from build123d import *

# Parameters (mm, degrees)
SKETCH1_W           = 47
SKETCH1_H           = 23.6
SKETCH1_W_2         = 44.18
SKETCH1_H_2         = 19
BOSS_EXTRUDE1_DEPTH = 5.5
SKETCH3_W           = 44.18
SKETCH3_H           = 19
BOSS_EXTRUDE2_DEPTH = 3
SKETCH6_W           = 7.25
SKETCH6_H           = 5.5
BOSS_EXTRUDE3_DEPTH = 5.25
SKETCH7_W           = 7.25
SKETCH7_H           = 5.5
BOSS_EXTRUDE4_DEPTH = 5.25
SKETCH8_R           = 1.5
CUT_EXTRUDE2_DEPTH  = 6.5
SKETCH9_W           = 51.734881385
SKETCH9_H           = 36.74917656
CUT_EXTRUDE3_DEPTH  = 3
SKETCH10_W          = 1.41
SKETCH10_H          = 14
BOSS_EXTRUDE5_DEPTH = 4
SKETCH11_W          = 3
SKETCH11_H          = 2.5
BOSS_EXTRUDE6_DEPTH = 3
SKETCH12_W          = 1.41
SKETCH12_H          = 8
CUT_EXTRUDE4_DEPTH  = 3.6
FILLET1_R           = 0.7


with BuildPart() as part:
    # Sketch1 → Boss-Extrude1 (new body)
    with BuildSketch(Plane(origin=(0, 0, 0), x_dir=(1, 0, 0), z_dir=(0, 1, 0))):
        with Locations((22.09, 9.5)):
            Rectangle(SKETCH1_W, SKETCH1_H)
        with Locations((22.09, 9.5)):
            Rectangle(SKETCH1_W_2, SKETCH1_H_2, mode=Mode.SUBTRACT)
    extrude(amount=BOSS_EXTRUDE1_DEPTH)

    # Sketch3 → Boss-Extrude2 (add)
    with BuildSketch(Plane.XZ):
        with Locations((22.09, -9.5)):
            Rectangle(SKETCH3_W, SKETCH3_H)
    extrude(amount=-BOSS_EXTRUDE2_DEPTH)

    # Sketch6 → Boss-Extrude3 (add)
    with BuildSketch(Plane.XY.offset(2.3)):
        with Locations((2.215, 2.75)):
            Rectangle(SKETCH6_W, SKETCH6_H)
        with Locations((41.965, 2.75)):
            Rectangle(SKETCH6_W, SKETCH6_H)
    extrude(amount=BOSS_EXTRUDE3_DEPTH)

    # Sketch7 → Boss-Extrude4 (add)
    with BuildSketch(Plane(origin=(0, 0, -21.3), x_dir=(-1, 0, 0), z_dir=(0, 0, -1))):
        with Locations((-41.965, 2.75)):
            Rectangle(SKETCH7_W, SKETCH7_H)
        with Locations((-2.215, 2.75)):
            Rectangle(SKETCH7_W, SKETCH7_H)
    extrude(amount=BOSS_EXTRUDE4_DEPTH)

    # Sketch8 → Cut-Extrude2 (cut, through all)
    with BuildSketch(Plane(origin=(0, 5.5, 0), x_dir=(1, 0, 0), z_dir=(0, 1, 0))):
        with Locations((41.965, 22.925)):
            Circle(SKETCH8_R)
        with Locations((41.965, -3.925)):
            Circle(SKETCH8_R)
        with Locations((2.215, -3.925)):
            Circle(SKETCH8_R)
        with Locations((2.215, 22.925)):
            Circle(SKETCH8_R)
    extrude(amount=-CUT_EXTRUDE2_DEPTH, mode=Mode.SUBTRACT)

    # Sketch9 → Cut-Extrude3 (cut)
    with BuildSketch(Plane.XZ):
        with Locations((23.178173587, -9.700906739)):
            Rectangle(SKETCH9_W, SKETCH9_H)
    extrude(amount=-CUT_EXTRUDE3_DEPTH, mode=Mode.SUBTRACT)

    # Sketch10 → Boss-Extrude5 (add)
    with BuildSketch(Plane(origin=(0, 5.5, 0), x_dir=(1, 0, 0), z_dir=(0, 1, 0))):
        with Locations((-0.705, 9.5)):
            Rectangle(SKETCH10_W, SKETCH10_H)
    extrude(amount=BOSS_EXTRUDE5_DEPTH)

    # Sketch11 → Boss-Extrude6 (add)
    with BuildSketch(Plane.ZY.offset(-44.18)):
        with Locations((-17.5, 4.25)):
            Rectangle(SKETCH11_W, SKETCH11_H)
        with Locations((-1.5, 4.25)):
            Rectangle(SKETCH11_W, SKETCH11_H)
    extrude(amount=BOSS_EXTRUDE6_DEPTH)

    # Sketch12 → Cut-Extrude4 (cut)
    with BuildSketch(Plane.XZ.offset(-3)):
        with Locations((-0.705, -9.5)):
            Rectangle(SKETCH12_W, SKETCH12_H)
    extrude(amount=-CUT_EXTRUDE4_DEPTH, mode=Mode.SUBTRACT)

    # Fillet1
    fillet1_edges = [part.edges().sort_by_distance(p)[0] for p in [
        (45.59, 5.5, -9.5),
        (0, 5.5, -17.75),
        (-1.41, 5.5, 2.525),
        (0, 5.5, -1.25),
        (20.59, 5.5, 0),
        (-1.41, 7.5, -16.5),
        (-0.705, 5.5, -2.5),
        (-1.41, 7.5, -2.5),
        (0, 7.5, -2.5),
        (-0.705, 5.5, -16.5),
        (0, 7.5, -16.5),
        (20.59, 5.5, -19),
        (42.68, 5.5, -16),
        (41.18, 5.5, -17.5),
        (44.18, 5.5, -9.5),
        (42.68, 5.5, -3),
        (41.18, 5.5, -1.5),
        (-1.41, 5.5, -21.525),
        (22.09, 5.5, 2.3),
        (5.84, 5.5, 4.925),
        (2.215, 5.5, 7.55),
        (38.34, 5.5, 4.925),
        (41.965, 5.5, 7.55),
        (22.09, 5.5, -21.3),
        (38.34, 5.5, -23.925),
        (41.965, 5.5, -26.55),
        (5.84, 5.5, -23.925),
        (2.215, 5.5, -26.55),
    ]]
    fillet(fillet1_edges, radius=FILLET1_R)


solid = part.part
Input: part model. Units: mm. Frame: model coordinates. A direction names the side the tool comes from. Give positions to 0.01 mm unless a question says otherwise; leave off trailing zeros. Write each loop counter-clockwise with the first axis right and the second up, starting at its lowest first coordinate (ties: lowest second). Pieces come first, ordered by that corner, then holes.
Q1. Section B-B, the plane x = 23. Output: boundary loops of the cut face in (y, z).
Q2. Set-up query: faces 4 (the face through (22, 4, 2.3)), 5 (the face through (43, 4, -3)), 6 (the face through (-1, 6.6, -9)). Return all of +Z, -Z, +X, -X, +Y, -Y with unobstructed straight access to the full face (end or side cutting, diameter ignored); none if empty.
Q3. Section C-C, the plane y = 3.75. Output: boundary loops of the cut face in (x, z) (3 decimals), plus the area to 3 significant figures.
Q4. Pull-direction query (X, two-part tool) for faces 1 (the face through (1.89, 4.27, -21.46)), 2 (the face through (-1, 9.5, -10)), 3 (the face through (0, 7, -9)); classes: pulls with the +X half, pulls with the -X half, needs draft (parallel to the pull), parting line crosses it, or undercut.
Q5. First-contact query: P1, Ø8, axis at x = 40, z = -9.5, coming from the -Y side; P2, Ø8, axis at x = 3.5, z = -7.5, coming from the -Y side; P3, Ø1, axis at y = 5.5, z = -0.5, coming from the +X side; P4, Ø1.4, axis at y = 4.5, z = -9, coming from the -X side. Flat tips, straight axial feed; report the tip coordinate or a pass-through.
Q6. Material intervals for probe 1 along X at (y, z) = (4.5, -17.5); probe 2 along X at (y, z) = (3.5, 4.5); probe 3 along X at (y, z) = (4, -5), sorted ascending.
Filled in:
1. outline: (3, -21.3) - (4.8, -21.3) arc R0.7 ccw to (5.5, -20.6) - (5.5, -19.7) arc R0.7 ccw to (4.8, -19) - (3, -19) - close; (3, 0) - (4.8, 0) arc R0.7 ccw to (5.5, 0.7) - (5.5, 1.6) arc R0.7 ccw to (4.8, 2.3) - (3, 2.3) - close
2. face 4: +Z, +Y, -Y
2. face 5: +Y, -Y
2. face 6: +X, -X, -Y
3. outline: (-1.41, -26.55) - (5.84, -26.55) - (5.84, -21.3) - (38.34, -21.3) - (38.34, -26.55) - (45.59, -26.55) - (45.59, 7.55) - (38.34, 7.55) - (38.34, 2.3) - (5.84, 2.3) - (5.84, 7.55) - (-1.41, 7.55) - (-1.41, -5.5) - (0, -5.5) - (0, 0) - (41.18, 0) - (41.18, -3) - (44.18, -3) - (44.18, -16) - (41.18, -16) - (41.18, -19) - (0, -19) - (0, -13.5) - (-1.41, -13.5) - close; hole circle Ø3 at (2.215, -22.925); hole circle Ø3 at (2.215, 3.925); hole circle Ø3 at (41.965, -22.925); hole circle Ø3 at (41.965, 3.925)
3. area: 400 mm2
4. face 1: undercut
4. face 2: needs draft
4. face 3: undercut
5. P1: passes through
5. P2: stops at y = 6.6
5. P3: stops at x = 45.56
5. P4: stops at x = 44.18
6. probe 1: x = -1.41 to 0, 41.18 to 45.59
6. probe 2: x = -1.41 to 0.83, 3.6 to 5.84, 38.34 to 40.58, 43.35 to 45.59
6. probe 3: x = -1.41 to 0, 44.18 to 45.59
